The listing builds one solid part. Answer for the finished solid, in the listing's coordinates (mm). Coordinates: 2 decimals unless noted, no trailing zeros. Order: outer loops, then holes, each group sorted by start corner. A loop starts at its lowest first (then second) coordinate and runs counter-clockwise, first axis right, second up.
from build123d import *

# Parameters (mm, degrees)
BOSS_EXTRUDE1_DEPTH = 5
FILLET1_R           = 25
SKETCH2_R           = 6
BOSS_EXTRUDE2_DEPTH = 153
FILLET2_R           = 10
FILLET3_R           = 10


with BuildPart() as part:
    # Sketch1 → Boss-Extrude1 (new, symmetric)
    with BuildSketch(Plane.XY):
        Polygon((-355, -107.5), (-385, -107.5), (-385, -77.5), (-355, -77.5), (-355, 107.5), (355, 107.5), (355, -77.5), (385, -77.5), (385, -107.5), (355, -107.5), align=None)
    extrude(amount=BOSS_EXTRUDE1_DEPTH, both=True)

    # Fillet1
    fillet1_edges = [part.edges().sort_by_distance(p)[0] for p in [
        (-355, -77.5, 0),
        (355, -77.5, 0),
    ]]
    fillet(fillet1_edges, radius=FILLET1_R)

    # Sketch2 → Boss-Extrude2 (add)
    with BuildSketch(Plane(origin=(0, 0, -5), x_dir=(-1, 0, 0), z_dir=(0, 0, -1))):
        with Locations(Location((-358, -90.5, 0), (0, 0, 180))):
            Circle(SKETCH2_R)
        with Locations(Location((358, -90.5, 0), (0, 0, 180))):
            Circle(SKETCH2_R)
    extrude(amount=BOSS_EXTRUDE2_DEPTH)

    # Fillet2
    fillet2_edges = [part.edges().sort_by_distance(p)[0] for p in [
        (-385, -107.5, 0),
        (385, -107.5, 0),
        (352, -90.5, -5),
        (-364, -90.5, -5),
    ]]
    fillet(fillet2_edges, radius=FILLET2_R)

    # Fillet3
    fillet3_edges = [part.edges().sort_by_distance(p)[0] for p in [
        (-385, -77.5, 0),
        (385, -77.5, 0),
    ]]
    fillet(fillet3_edges, radius=FILLET3_R)


solid = part.part
(1) Find section C-C on x = -175.5. Determine the outline of the cut face in (y, z).
(2) Find the intervals of material crossed by probe 1 along Z at (x, y) = (-257, 46.5); probe 2 along X at (y, z) = (-86.5, -76.5), in increasing order.
(3) Given pin 1 Ø3 at (x, y) = (114, -26) entering from -Z; pin 2 Ø3 at (y, z) = (5, 0) entering from +X; pin 3 Ø5 at (y, z) = (57, 1) entering from -X, each flat-ended and moving along its own axis, determine where each tip first touches the part or whether it passes through.
(4) Find section B-B on y = -35. Determine the outline of the cut face in (x, z), then the cut area to 3 significant figures.
(5) Find section A-A on z = -59. Determine the outline of the cut face in (x, y), then the cut area to 3 significant figures.
Resolved:
1. outline: (-107.5, -5) - (107.5, -5) - (107.5, 5) - (-107.5, 5) - close
2. probe 1: z = -5 to 5
2. probe 2: x = -362.47 to -353.53, 353.53 to 362.47
3. pin 1: stops at z = -5
3. pin 2: stops at x = 355
3. pin 3: stops at x = -355
4. outline: (-355, -5) - (355, -5) - (355, 5) - (-355, 5) - close
4. area: 7,100 mm2
5. outline: circle Ø12 at (-358, -90.5); circle Ø12 at (358, -90.5)
5. area: 226 mm2
